Read the model definition and answer for the solid it produces. Units are mm, in the model's axes. A direction names the side the tool comes from. Coordinates: 2 decimals unless noted, no trailing zeros. Order: outer loops, then holes, each group sorted by start corner. A loop starts at its lowest first (then second) coordinate and runs counter-clockwise, first axis right, second up.
from build123d import *

# Parameters (mm, degrees)
SKETCH1_R           = 1
BOSS_EXTRUDE1_DEPTH = 3
SKETCH1_3_R         = 0.5
BOSS_EXTRUDE2_DEPTH = 1.5


with BuildPart() as part:
    # Sketch1 → Boss-Extrude1 (new body)
    with BuildSketch(Plane(origin=(0, 0, 0), x_dir=(1, 0, 0), z_dir=(0, 1, 0))):
        with BuildLine():
            ThreePointArc((-46.139075952, 38.780795182), (-35.068281039, 36.285100261), (-26.139075952, 29.280795182))
            Line((-26.139075952, 29.280795182), (-23.139075952, 29.280795182))
            Line((-23.139075952, 29.280795182), (-23.139075952, 59.280795182))
            Line((-23.139075952, 59.280795182), (-26.139075952, 59.280795182))
            ThreePointArc((-26.139075952, 59.280795182), (-35.068281039, 52.276490103), (-46.139075952, 49.780795182))
            ThreePointArc((-46.139075952, 49.780795182), (-51.639075952, 44.280795182), (-46.139075952, 38.780795182))
        make_face()
        with BuildLine():
            ThreePointArc((-43.42430156, 41.480795182), (-50.039075952, 44.280795182), (-43.42430156, 47.080795182))
            Line((-43.42430156, 47.080795182), (-31.023874876, 46.380795182))
            ThreePointArc((-31.023874876, 46.380795182), (-29.039075952, 44.280795182), (-31.023874876, 42.180795182))
            Line((-31.023874876, 42.180795182), (-43.42430156, 41.480795182))
        make_face(mode=Mode.SUBTRACT)
        with Locations(Location((-24.639075952, 54.280795182, 0), (0, 0, 270))):
            Circle(SKETCH1_R, mode=Mode.SUBTRACT)
        with Locations(Location((-24.639075952, 34.280795182, 0), (0, 0, 270))):
            Circle(SKETCH1_R, mode=Mode.SUBTRACT)
    extrude(amount=-BOSS_EXTRUDE1_DEPTH)

    # Sketch1_3 → Boss-Extrude2 (add)
    with BuildSketch(Plane(origin=(0, 0, 0), x_dir=(1, 0, 0), z_dir=(0, 1, 0))):
        with BuildLine():
            ThreePointArc((-43.42430156, 47.080795182), (-42.239075952, 44.280795182), (-43.42430156, 41.480795182))
            Line((-43.42430156, 41.480795182), (-31.023874876, 42.180795182))
            ThreePointArc((-31.023874876, 42.180795182), (-29.039075952, 44.280795182), (-31.023874876, 46.380795182))
            Line((-31.023874876, 46.380795182), (-43.42430156, 47.080795182))
        make_face()
        with Locations(Location((-41.023874876, 44.280795182, 0), (0, 0, 270))):
            Circle(SKETCH1_3_R, mode=Mode.SUBTRACT)
        with Locations(Location((-33.023874876, 44.280795182, 0), (0, 0, 270))):
            Circle(SKETCH1_3_R, mode=Mode.SUBTRACT)
        with Locations(Location((-31.023874876, 44.280795182, 0), (0, 0, 270))):
            Circle(SKETCH1_3_R, mode=Mode.SUBTRACT)
        with Locations(Location((-39.023874876, 44.280795182, 0), (0, 0, 270))):
            Circle(SKETCH1_3_R, mode=Mode.SUBTRACT)
        with Locations(Location((-37.023874876, 44.280795182, 0), (0, 0, 270))):
            Circle(SKETCH1_3_R, mode=Mode.SUBTRACT)
        with Locations(Location((-35.023874876, 44.280795182, 0), (0, 0, 270))):
            Circle(SKETCH1_3_R, mode=Mode.SUBTRACT)
    extrude(amount=-BOSS_EXTRUDE2_DEPTH)


solid = part.part
Q1. The part is cut by section D-D, the plane z = -40.75. Determine the outline of the cut face in (x, y).
Q2. Straight lines are drawn through the part: L1, parallel to Z at x = -24.25, y = -1.2; L2, parallel to Z at x = -32.75, y = -1.3; L3, parallel to X at y = -1.3, z = -42. For each, find the intervals that lie inside material, in ascending order.
Q3. The part is cut by section A-A, the plane z = -54.75. Determine the outline of the cut face in (x, y).
Q4. The part is cut by section B-B, the plane y = -1.9. Determine the outline of the cut face in (x, z).
Q5. Determine the mould class of faces 1 (the cylindrical face through (-51.638, -1.479, -44.402)), 2 (the flat face through (-23.139, -1, -44)), 3 (the cylindrical face through (-25.526, -1.479, -33.819)) for opening direction Z: +Z half, -Z half, draft (parallel to the pull), parting line (faces both ways), or undercut.
Q6. The part is cut by section C-C, the plane x = -42.75. Determine the outline of the cut face in (y, z).
Q7. Which of the six approach directions +Z, -Z, +X, -X, +Y, -Y give full straight-line access (tool end or side, diameter ignored) to faces 4 (the flat face through (-25, -1, -59.281)), 5 (the flat face through (-37.137, -2.24, -41.836))?
Q8. Each of these flat-tipped pins is pushed along its axis until it touches: P1, Ø1.6, axis at x = -24.64, z = -34.28, coming from the -Y side; P2, Ø1, axis at x = -47.5, y = -1, coming from the -Z side. Where does it stop, or does it pass through?
Computed values:
1. outline: (-50.36, -3) - (-47.8, -3) - (-47.8, 0) - (-50.36, 0) - close; (-44.48, -3) - (-23.14, -3) - (-23.14, 0) - (-44.48, 0) - close
2. L1: z = -59.28 to -55.2, -53.36 to -35.2, -33.36 to -29.28
2. L2: z = -53.53 to -44.7, -43.86 to -35.04
2. L3: x = -51.14 to -49.3, -42.98 to -23.14
3. outline: (-30.92, -3) - (-25.52, -3) - (-25.52, 0) - (-30.92, 0) - close; (-23.76, -3) - (-23.14, -3) - (-23.14, 0) - (-23.76, 0) - close
4. outline: (-46.14, -49.78) arc R25.8 cw to (-26.14, -59.28) - (-23.14, -59.28) - (-23.14, -29.28) - (-26.14, -29.28) arc R25.8 cw to (-46.14, -38.78) arc R5.5 ccw to start; hole (-43.42, -47.08) - (-31.02, -46.38) arc R2.1 ccw to (-31.02, -42.18) - (-43.42, -41.48) arc R3.9 ccw (long way) to start; hole circle Ø2 at (-24.64, -54.28); hole circle Ø2 at (-24.64, -34.28)
5. face 1: parting line
5. face 2: draft
5. face 3: undercut
6. outline: (-3, -50) - (0, -50) - (0, -46.21) - (-1.5, -46.21) - (-1.5, -47.04) - (-3, -47.04) - close; (-3, -41.52) - (-1.5, -41.52) - (-1.5, -42.35) - (0, -42.35) - (0, -38.56) - (-3, -38.56) - close
7. face 4: -Z, +X, -X, +Y, -Y
7. face 5: -Y
8. P1: passes through
8. P2: stops at z = -49.71
